Here's how the part is built. I have some questions about the finished solid (model axes, mm). Coordinates: 2 decimals unless noted, no trailing zeros. Loops run counter-clockwise (first coordinate to the right, second up) from the corner with the lowest first, then second, coordinate; pieces in that order, holes last. Notation, with made-up numbers: (-32, -6.5) -> (27, -6.5) arc R23 cw to (27, 19.5) -> close; hole circle Ø11 at (-21.5, 85.25). An arc over 180 degrees is marked (long way). Answer as a JSON object with one key per item and string values. Group by question number.
1) I want a section at D-D (y = -8.25). Write out the boundary of the cut face in (x, z), then the cut area to 3 significant figures.
2) I want a section at A-A (y = -4.25). Write out the boundary of the cut face in (x, z), then the cut area to 3 significant figures.
3) I want a section at C-C (x = 62). Write out the boundary of the cut face in (y, z).
4) I need wall thicknesses on probe 1 along Z at (x, y) = (0, -2.25); probe 2 along Z at (x, y) = (0, -7.5); probe 3 along Y at (x, z) = (-1, 44). Which ranges of each line are inside material? Lowest first, please. Write a range as [from, to].
5) I'm going to push flat-ended pins straight in: pin 1 (5 mm diameter, centred on y = -6, z = 24, fed in from +X); pin 2 (3 mm diameter, centred on x = 21, y = -2, fed in from -Z); pin 3 (1.5 mm diameter, centred on x = 60.5, y = -6.5, fed in from -Z); pin 4 (2 mm diameter, centred on x = 42.5, y = -7.5, fed in from +Z). Where does each tip first touch, or does it pass through?
6) I want a section at B-B (x = 2). Write out the boundary of the cut face in (y, z) (3 decimals), then the cut area to 3 significant figures.
```python
from build123d import *

# Parameters (mm, degrees)
F0_R     = 3.81
F1_DEPTH = 6.35
F2_R     = 3.81
F3_DEPTH = 3.175


# Not quite as in the source:
# - a feature names something its author has since deleted; it is built from what else it names


with BuildPart() as f1:
    # F0 (on Front) → F1 (new body)
    with BuildSketch(Plane.XZ):
        with BuildLine():
            ThreePointArc((64.087961787, 5.2589050049), (58.2083291, 0), (64.087961787, -5.2589050049))
            ThreePointArc((64.087961787, -5.2589050049), (67.4441780635, -3.5277812174), (68.7916709, 0))
            ThreePointArc((68.7916709, 0), (67.4441780635, 3.5277812174), (64.087961787, 5.2589050049))
        make_face()
        with Locations((63.5, 0)):
            Circle(F0_R, mode=Mode.SUBTRACT)
        with BuildLine():
            ThreePointArc((5.2589006137, 64.087962963), (5.2834688034, 63.794437625), (5.2916666667, 63.5))
            ThreePointArc((5.2916666667, 63.5), (0, 58.2083333333), (-5.2916666667, 63.5))
            Line((-5.2916666667, 63.5), (-8.7637923714, 32.7392136171))
            ThreePointArc((-8.7637923714, 32.7392136171), (0.0046668449, 40.5694432097), (8.7648343562, 32.7299382716))
            Line((8.7648343562, 32.7299382716), (5.2589006137, 64.087962963))
        make_face()
        with BuildLine():
            ThreePointArc((-5.2916666667, 63.5), (0, 58.2083333333), (5.2916666667, 63.5))
            ThreePointArc((5.2916666667, 63.5), (5.2834688034, 63.794437625), (5.2589006137, 64.087962963))
            ThreePointArc((5.2589006137, 64.087962963), (-0.294437625, 68.7834688034), (-5.2916666667, 63.5))
        make_face()
        with Locations((0, 63.5)):
            Circle(F0_R, mode=Mode.SUBTRACT)
        with BuildLine():
            ThreePointArc((8.8131488161, 31.4168209877), (0, 22.9305555556), (-8.8131488161, 31.4168209877))
            Line((-8.8131488161, 31.4168209877), (-7.6145605771, -0.2878666667))
            ThreePointArc((-7.6145605771, -0.2878666667), (-0.1439590264, 7.6186400229), (7.62, 0))
            ThreePointArc((7.62, 0), (5.3881536726, -5.3881536726), (0, -7.62))
            Line((0, -7.62), (31.4152979668, -8.8130854583))
            ThreePointArc((31.4152979668, -8.8130854583), (22.9364968819, -0.3235174392), (30.7700650994, 8.7648290535))
            Line((30.7700650994, 8.7648290535), (29.8488925204, 8.6618391202))
            ThreePointArc((29.8488925204, 8.6618391202), (14.7662444168, 13.637318243), (8.6958303376, 28.313548659))
            Line((8.6958303376, 28.313548659), (8.8131488161, 31.4168209877))
        make_face()
        with BuildLine():
            ThreePointArc((30.7700650994, 8.7648290535), (22.9364968819, -0.3235174392), (31.4152979668, -8.8130854583))
            ThreePointArc((31.4152979668, -8.8130854583), (32.0735174392, -8.8135031181), (32.7299349006, -8.7648290535))
            ThreePointArc((32.7299349006, -8.7648290535), (38.3236206398, -5.8796268956), (40.5694388, 0))
            ThreePointArc((40.5694388, 0), (38.3236206398, 5.8796268956), (32.7299349006, 8.7648290535))
            ThreePointArc((32.7299349006, 8.7648290535), (31.75, 8.8194388), (30.7700650994, 8.7648290535))
        make_face()
        with BuildLine():
            ThreePointArc((40.5694388, 0), (38.3236206398, -5.8796268956), (32.7299349006, -8.7648290535))
            Line((32.7299349006, -8.7648290535), (64.087961787, -5.2589050049))
            ThreePointArc((64.087961787, -5.2589050049), (58.2083291, 0), (64.087961787, 5.2589050049))
            Line((64.087961787, 5.2589050049), (32.7299349006, 8.7648290535))
            ThreePointArc((32.7299349006, 8.7648290535), (38.3236206398, 5.8796268956), (40.5694388, 0))
        make_face()
        with BuildLine():
            ThreePointArc((7.62, 0), (-0.1439590264, 7.6186400229), (-7.6145605771, -0.2878666667))
            ThreePointArc((-7.6145605771, -0.2878666667), (-5.2853976199, -5.4889864274), (0, -7.62))
            ThreePointArc((0, -7.62), (5.3881536726, -5.3881536726), (7.62, 0))
        make_face()
        Circle(F0_R, mode=Mode.SUBTRACT)
        with BuildLine():
            ThreePointArc((8.8194444444, 31.75), (8.8057813389, 32.240729375), (8.7648343562, 32.7299382716))
            ThreePointArc((8.7648343562, 32.7299382716), (0.0046668449, 40.5694432097), (-8.7637923714, 32.7392136171))
            ThreePointArc((-8.7637923714, 32.7392136171), (-8.8133078888, 32.0789443195), (-8.8131488161, 31.4168209877))
            ThreePointArc((-8.8131488161, 31.4168209877), (0, 22.9305555556), (8.8131488161, 31.4168209877))
            ThreePointArc((8.8131488161, 31.4168209877), (8.8178703969, 31.5833807565), (8.8194444444, 31.75))
        make_face()
    extrude(amount=F1_DEPTH)

    # F2 (on face) → F3 (join)
    with BuildSketch(Plane.XZ.offset(6.35)):
        with BuildLine():
            ThreePointArc((0, -7.62), (5.3881536726, -5.3881536726), (7.62, 0))
            ThreePointArc((7.62, 0), (-0.1439590264, 7.6186400229), (-7.6145605771, -0.2878666667))
            ThreePointArc((-7.6145605771, -0.2878666667), (-5.2853976199, -5.4889864274), (0, -7.62))
        make_face()
        Circle(F2_R, mode=Mode.SUBTRACT)
    extrude(amount=F3_DEPTH)


solid = f1.part
```
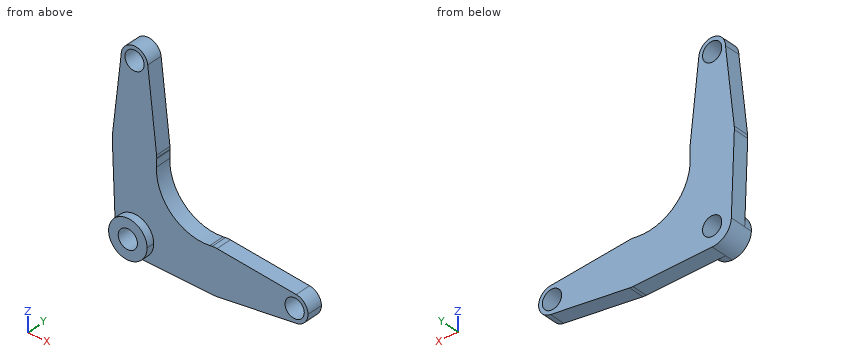
Determined:
{
 "1": {"outline": "circle Ø15.24 at (0, 0); hole circle Ø7.62 at (0, 0)", "area": "137 mm^2"},
 "2": {"outline": "(-8.81, 31.42) -> (-7.61, -0.29) arc R7.62 ccw to (0, -7.62) -> (31.42, -8.81) arc R8.82 ccw to (32.73, -8.76) -> (64.09, -5.26) arc R5.29 ccw to (64.09, 5.26) -> (32.73, 8.76) arc R8.82 ccw to (30.77, 8.76) -> (29.85, 8.66) arc R19.05 cw to (8.7, 28.31) -> (8.81, 31.42) arc R8.82 ccw to (8.76, 32.73) -> (5.26, 64.09) arc R5.29 ccw to (-5.29, 63.5) -> (-8.76, 32.74) arc R8.82 ccw to start; hole circle Ø7.62 at (0, 0); hole circle Ø7.62 at (0, 63.5); hole circle Ø7.62 at (63.5, 0)", "area": "1,970 mm^2"},
 "3": {"outline": "(-6.35, -5.49) -> (0, -5.49) -> (0, -3.5) -> (-6.35, -3.5) -> close; (-6.35, 3.5) -> (0, 3.5) -> (0, 5.49) -> (-6.35, 5.49) -> close"},
 "4": {"probe 1": "[-7.62, -3.81], [3.81, 59.69], [67.31, 68.79]", "probe 2": "[-7.62, -3.81], [3.81, 7.62]", "probe 3": "[-6.35, 0]"},
 "5": {"pin 1": "x = 9.68", "pin 2": "z = -8.47", "pin 3": "z = -5.74", "pin 4": "through"},
 "6": {"outline": "(-9.525, -7.353) -> (-6.35, -7.353) -> (-6.35, -7.696) -> (0, -7.696) -> (0, -3.243) -> (-9.525, -3.243) -> close; (-9.525, 3.243) -> (0, 3.243) -> (0, 60.257) -> (-6.35, 60.257) -> (-6.35, 7.353) -> (-9.525, 7.353) -> close; (-6.35, 66.743) -> (0, 66.743) -> (0, 68.399) -> (-6.35, 68.399) -> close", "area": "427 mm^2"}
}
